Part print with two shaded views. Sizes in mm from the minimum x, y, z corner. A direction names the side the tool comes from. Coordinates: 2 decimals unless noted, no trailing zeros. Loops run counter-clockwise (first coordinate to the right, second up) from the corner with the lowest first, then second, coordinate; pieces in that order, holes last. Notation, with made-up numbers: (63.5, 1.25) -> (98.5, 1.25) arc R31 ccw to (98.5, 35.25) -> close; hole circle Ø9 at (6.5, -12). An arc over 180 degrees is marked (long way). Write each question's results on one line, items separated by ' | '.
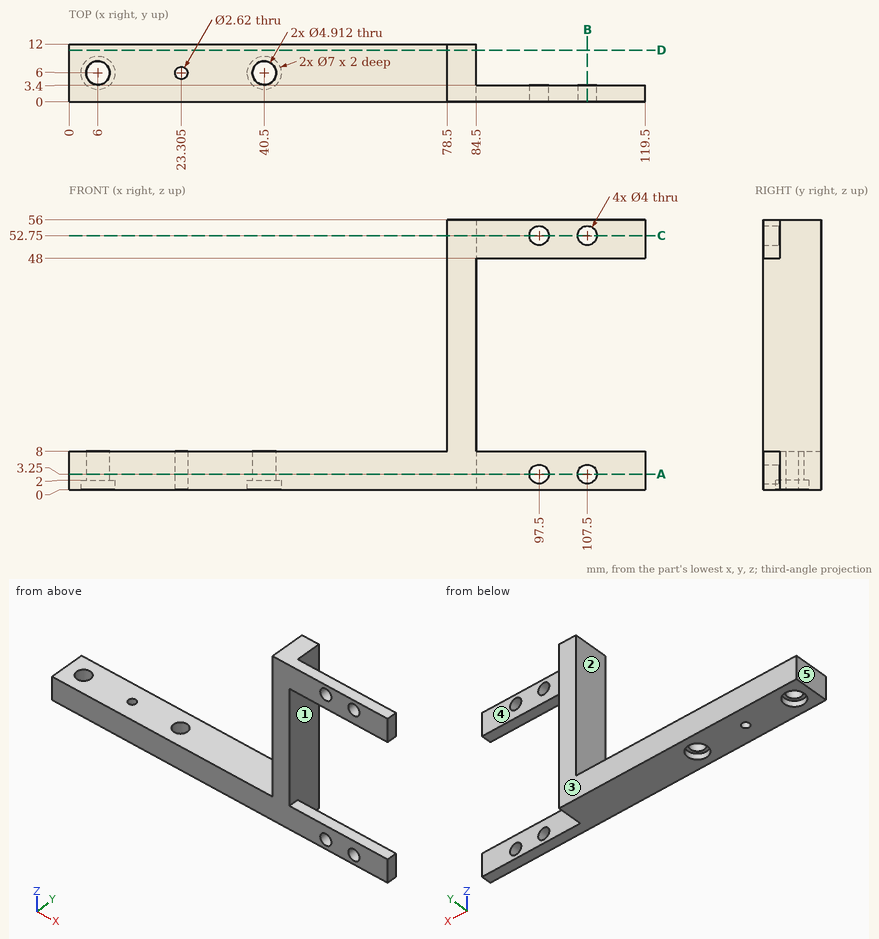
Q1. Cut at A-A on z = 3.25. Write the cut outline in (x, y) (1 decimal), and give its area (3 significant figures).
Results are:
outline: (0, 0) -> (95.5, 0) -> (95.5, 3.4) -> (84.5, 3.4) -> (84.5, 12) -> (0, 12) -> close; (99.5, 0) -> (105.5, 0) -> (105.5, 3.4) -> (99.5, 3.4) -> close; (109.5, 0) -> (119.5, 0) -> (119.5, 3.4) -> (109.5, 3.4) -> close; hole circle Ø4.9 at (6, 6); hole circle Ø2.6 at (23.3, 6); hole circle Ø4.9 at (40.5, 6) | area: 1,060 mm^2
Q2. Wall check: L1, parallel to Z at x = 107.5, y = 2.55; L2, parallel to Y at x = 6, z = 1.05; L3, parallel to Z at x = 26, y = 2. Give the ranges that are in metal, low to high. Write a range as from..to.
Results are:
L1: 0..1.25, 5.25..8, 48..50.75, 54.75..56 | L2: 0..2.5, 9.5..12 | L3: 0..8
Q3. Drop flat-ended pins along their axis: pin 1 (6 mm diameter, centred on x = 39, y = 5, fed in from +Z); pin 2 (6.5 mm diameter, centred on x = 107.5, z = 52.75, fed in from +Y). Give the stop position or say it passes through.
Results are:
pin 1: z = 8 | pin 2: y = 3.4
Q4. Cut at D-D on y = 10.75. Write the cut outline in (x, z), and give its area (3 significant figures).
Results are:
outline: (0, 0) -> (84.5, 0) -> (84.5, 56) -> (78.5, 56) -> (78.5, 8) -> (0, 8) -> close | area: 964 mm^2
Q5. Cut at C-C on z = 52.75. Write the cut outline in (x, y), and give its area (3 significant figures).
Results are:
outline: (78.5, 0) -> (95.5, 0) -> (95.5, 3.4) -> (84.5, 3.4) -> (84.5, 12) -> (78.5, 12) -> close; (99.5, 0) -> (105.5, 0) -> (105.5, 3.4) -> (99.5, 3.4) -> close; (109.5, 0) -> (119.5, 0) -> (119.5, 3.4) -> (109.5, 3.4) -> close | area: 164 mm^2
Q6. Cut at B-B on x = 107.5. Write the cut outline in (y, z).
Results are:
outline: (0, 0) -> (3.4, 0) -> (3.4, 1.25) -> (0, 1.25) -> close; (0, 5.25) -> (3.4, 5.25) -> (3.4, 8) -> (0, 8) -> close; (0, 48) -> (3.4, 48) -> (3.4, 50.75) -> (0, 50.75) -> close; (0, 54.75) -> (3.4, 54.75) -> (3.4, 56) -> (0, 56) -> close
Q7. Which spindle directions (+Z, -Z, +X, -X, +Y, -Y) get a long thin tool onto all of the face, cutting with end or side? Do the marked faces 1, 2, 3, 4 and 5. Say none if no direction does.
Results are:
face 1: +X, +Y | face 2: +Z, -X, +Y, -Y | face 3: +Z, -Z, +X, -X, +Y | face 4: +Z, -Z, +X, +Y | face 5: +Z, -Z, -X, +Y, -Y
